Read the model definition and answer for the solid it produces. Units are mm, in the model's axes. Coordinates: 2 decimals unless noted, no trailing zeros. Write each loop counter-clockwise with the first axis right and the second up, starting at its lowest first coordinate (ties: lowest second). Pieces come first, ordered by that corner, then holes. Notation, with made-up numbers: (75.5, 29) -> (88.5, 29) arc R15 ccw to (88.5, 43) -> close; hole circle Ø2 at (-28.5, 55.25). An arc over 180 degrees is marked (long way). Answer in a Markdown table with one row per item. Add a question column.
Item 1: Section C-C on y = 7 is taken. Write down the section's boundary in (x, z) (1 decimal).
Item 2: Given pin 1 Ø6 at (y, z) = (25, -129) entering from +X (3 decimals); pin 2 Ø10 at (y, z) = (11, 24) entering from +X (3 decimals); pin 3 Ø12 at (x, y) = (168, 29.5) entering from -Z (3 decimals), each flat-ended and moving along its own axis, determine where each tip first touches the part or whether it passes through.
Item 3: Straight lines are drawn through the part: line 1 (Z direction, x = -278, y = 20.5) (3 decimals); line 2 (Z direction, x = -247, y = 27.5) (3 decimals); line 3 (X direction, y = 8, z = -15.5) (3 decimals). For each, find the intervals that lie inside material, in ascending order. Write a range as from..to.
Item 4: Section D-D on x = 164 is taken. Write down the section's boundary in (y, z) (3 decimals), then the cut area to 3 significant figures.
Item 5: Section A-A on x = -238.5 is taken. Write down the section's boundary in (y, z) (3 decimals), then the cut area to 3 significant figures.
Item 6: Section B-B on z = 20 is taken. Write down the section's boundary in (x, y) (3 decimals), then the cut area to 3 significant figures.
Item 7: For a pull along Z with two mould halves and no side action, classify faces 1 (the face through (-246, 19, -294.305)), 2 (the face through (5, 19, 294.305)), 3 (the face through (-281.44, 18.78, 46.32)) as +Z half, -Z half, draft (parallel to the pull), parting line (faces both ways), or undercut.
```python
from build123d import *

# Parameters (mm, degrees)
BOSS_EXTRUDE1_DEPTH = 38.1
SKETCH2_R           = 27
CUT_EXTRUDE1_DEPTH  = 39.1


with BuildPart() as part:
    # Sketch1 → Boss-Extrude1 (new body)
    with BuildSketch(Plane(origin=(0, 0, 0), x_dir=(1, 0, 0), z_dir=(0, 1, 0))):
        Polygon((-138.61, 294.305), (350, -194.305), (350, -294.305), (-350, -294.305), (-350, 294.305), align=None)
    extrude(amount=BOSS_EXTRUDE1_DEPTH)

    # Sketch2 → Cut-Extrude1 (cut, through all)
    with BuildSketch(Plane(origin=(0, 0, 0), x_dir=(-1, 0, 0), z_dir=(0, -1, 0))):
        with Locations((256.500204402, -35.980503112)):
            Circle(SKETCH2_R)
    extrude(amount=-CUT_EXTRUDE1_DEPTH, mode=Mode.SUBTRACT)


solid = part.part
```
Results below:
| question | item | result |
|---|---|---|
| 1 | outline | (-350, -294.3) -> (-138.6, -294.3) -> (350, 194.3) -> (350, 294.3) -> (-350, 294.3) -> close; hole circle Ø54 at (-256.5, 36) |
| 2 | pin 1 | stops at x = 29.695 |
| 2 | pin 2 | stops at x = 184.695 |
| 2 | pin 3 | stops at z = 6.305 |
| 3 | line 1 | z = -294.305..19.648, 52.313..294.305 |
| 3 | line 2 | z = -294.305..10.707, 61.254..294.305 |
| 3 | line 3 | x = -350..140.195 |
| 4 | outline | (0, 8.305) -> (38.1, 8.305) -> (38.1, 294.305) -> (0, 294.305) -> close |
| 4 | area | 10,900 mm2 |
| 5 | outline | (0, -294.305) -> (38.1, -294.305) -> (38.1, 15.856) -> (0, 15.856) -> close; (0, 56.105) -> (38.1, 56.105) -> (38.1, 294.305) -> (0, 294.305) -> close |
| 5 | area | 20,900 mm2 |
| 6 | outline | (-350, 0) -> (-278.263, 0) -> (-278.263, 38.1) -> (-350, 38.1) -> close; (-234.737, 0) -> (175.695, 0) -> (175.695, 38.1) -> (-234.737, 38.1) -> close |
| 6 | area | 18,400 mm2 |
| 7 | face 1 | -Z half |
| 7 | face 2 | +Z half |
| 7 | face 3 | undercut |
